Design review of the part built by this model. Coordinates are the model's own, in mm. Face numbers are marked on the shaded views. A direction names the side the tool comes from. Round coordinates to 2 decimals unless told otherwise and drop trailing zeros. Order: outer loops, then holes, each group sorted by start corner. A loop starts at its lowest first (then second) coordinate and runs counter-clockwise, first axis right, second up. Notation, with made-up numbers: (-40, -19.75) - (-25, -19.75) arc R34 cw to (-25, 16.25) - close; hole circle Ø5 at (-7.5, 51). An arc over 180 degrees is marked (long way). Write item = value, one per line.
from build123d import *

# Parameters (mm, degrees)
SKETCH_1_R                = 12
EXTRUDE_1_DEPTH           = 12
SKETCH_1_4_R              = 0.85
CUT_EXTRUDE_2_DEPTH       = 2.5
SKETCH_1_5_R              = 4
EXTRUDE_2_DEPTH           = 4
SKETCH_1_6_R              = 4.3
EXTRUDE_3_DEPTH           = 0.5
SKETCH_1_7_R              = 2
CUT_EXTRUDE_3_DEPTH       = 4
SKETCH_1_8_R              = 1.5
CUT_EXTRUDE_5_DEPTH       = 1
CUT_EXTRUDE_START         = 12
SKETCH_1_10_R             = 9
CUT_EXTRUDE_6_DEPTH       = 9.5
EXTRUDE_8_DEPTH           = 0.3
EXTRUDE_8_DEPTH_BACK      = 2.2
CUT_EXTRUDE_START_2       = -2.2
CUT_EXTRUDE_20_DEPTH      = 1.5
CUT_EXTRUDE_21_DEPTH      = 1
CUT_EXTRUDE_21_DEPTH_BACK = 2
SKETCH_3_10_R             = 0.85
FILLET_3_R                = 1.1


with BuildPart() as part:
    # 草图1 → 凸台-拉伸1 (new body)
    with BuildSketch(Plane.XY):
        Circle(SKETCH_1_R)
    extrude(amount=EXTRUDE_1_DEPTH)

    # 草图1<4> → 切除-拉伸2 (cut)
    with BuildSketch(Plane.XY):
        with Locations((0, 6)):
            Circle(SKETCH_1_4_R)
        with Locations((-5.196152423, -3)):
            Circle(SKETCH_1_4_R)
        with Locations(Location((5.196152423, -3, 0), (0, 0, 180))):
            Circle(SKETCH_1_4_R)
    extrude(amount=CUT_EXTRUDE_2_DEPTH, mode=Mode.SUBTRACT)

    # 草图1<5> → 凸台-拉伸2 (add)
    with BuildSketch(Plane.XY):
        Circle(SKETCH_1_5_R)
    extrude(amount=-EXTRUDE_2_DEPTH)

    # 草图1<6> → 凸台-拉伸3 (add)
    with BuildSketch(Plane.XY):
        Circle(SKETCH_1_6_R)
    extrude(amount=-EXTRUDE_3_DEPTH)

    # 草图1<7> → 切除-拉伸3 (cut)
    with BuildSketch(Plane.XY):
        Circle(SKETCH_1_7_R)
    extrude(amount=-CUT_EXTRUDE_3_DEPTH, mode=Mode.SUBTRACT)

    # 草图1<8> → 切除-拉伸5 (cut)
    with BuildSketch(Plane.XY):
        with Locations((-5.196152423, -3)):
            Circle(SKETCH_1_8_R)
        with Locations((5.196152423, -3)):
            Circle(SKETCH_1_8_R)
        with Locations((0, 6)):
            Circle(SKETCH_1_8_R)
    extrude(amount=CUT_EXTRUDE_5_DEPTH, mode=Mode.SUBTRACT)

    # 草图1<10> → 切除-拉伸6 (cut)
    with BuildSketch(Plane.XY.offset(CUT_EXTRUDE_START)):
        Circle(SKETCH_1_10_R)
    extrude(amount=-CUT_EXTRUDE_6_DEPTH, mode=Mode.SUBTRACT)

    # 草图3 → 凸台-拉伸8 (add, two sides: drawn at the far end of the back side and taken through both)
    with BuildSketch(Plane(origin=(14, 0, 0), x_dir=(0, 0, -1), z_dir=(1, 0, 0)).offset(-EXTRUDE_8_DEPTH_BACK)):
        Polygon((-18, -3), (-12, -3), (-6, -3), (-6, 3), (-18, 3), align=None)
        Polygon((-6, 3), (-6, -3), (0, -3), (6, -3), (6, 3), align=None)
    extrude(amount=EXTRUDE_8_DEPTH + EXTRUDE_8_DEPTH_BACK)

    # 草图3<9> → 切除-拉伸20 (cut)
    with BuildSketch(Plane(origin=(14, 0, 0), x_dir=(0, 0, -1), z_dir=(1, 0, 0)).offset(CUT_EXTRUDE_START_2)):
        Polygon((-13.130266283, 0), (-14.097327984, 1.675), (-16.031451386, 1.675), (-16.998513087, 0), (-16.031451386, -1.675), (-14.097327984, -1.675), align=None)
        Polygon((1.130266283, 0), (2.097327984, 1.675), (4.031451386, 1.675), (4.998513087, 0), (4.031451386, -1.675), (2.097327984, -1.675), align=None)
    extrude(amount=CUT_EXTRUDE_20_DEPTH, mode=Mode.SUBTRACT)

    # 草图3<10> → 切除-拉伸21 (cut, two sides: drawn at the far end of the back side and taken through both)
    with BuildSketch(Plane(origin=(14, 0, 0), x_dir=(0, 0, -1), z_dir=(1, 0, 0)).offset(-CUT_EXTRUDE_21_DEPTH_BACK)):
        with Locations(Location((3.064389685, 0, 0), (0, 0, 180))):
            Circle(SKETCH_3_10_R)
        with Locations(Location((-15.064389685, 0, 0), (0, 0, 180))):
            Circle(SKETCH_3_10_R)
    extrude(amount=CUT_EXTRUDE_21_DEPTH + CUT_EXTRUDE_21_DEPTH_BACK, mode=Mode.SUBTRACT)

    # 圆角3
    fillet_3_edges = [part.edges().sort_by_distance(p)[0] for p in [
        (13.05, 3, 18),
        (13.05, -3, 18),
        (13.05, 3, -6),
        (13.05, -3, -6),
    ]]
    fillet(fillet_3_edges, radius=FILLET_3_R)


solid = part.part
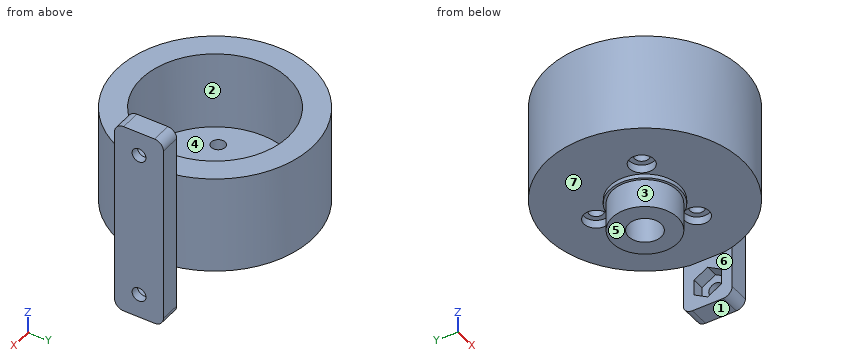
1) We need section C-C on z = 8.75. Write out the cut boundary in (x, y), and give its area (3 significant figures).
Findings:
outline = (11.8, -3) - (14.3, -3) - (14.3, 3) - (11.8, 3) - (11.8, 2.18) arc R12 ccw (long way) to (11.8, -2.18) - close; hole circle Ø18 at (0, 0)
area = 212 mm^2
2) We need section D-D on y = -10. Write out the cut boundary in (x, z).
Findings:
outline = (-6.63, 0) - (6.63, 0) - (6.63, 12) - (-6.63, 12) - close
3) Clearance check with flat-ended pins moving along their axes: pin 1 Ø1.5 at (x, y) = (0, 6.5) entering from -Z; pin 2 Ø10 at (y, z) = (-6.5, -2.5) entering from -X; pin 3 Ø4 at (x, z) = (-8, -1.5) entering from +Y. State where each tip first meets the part, or that it passes through.
Findings:
pin_1 = 1
pin_2 = -11.8
pin_3 = 9.97
4) We need section B-B on x = 8. Write out the cut boundary in (y, z), and give its area (3 significant figures).
Findings:
outline = (-8.94, 0) - (8.94, 0) - (8.94, 12) - (4.12, 12) - (4.12, 2.5) - (-4.12, 2.5) - (-4.12, 12) - (-8.94, 12) - close
area = 136 mm^2
5) To check wall thickness, follow L1, parallel to Y at x = 0, z = -0.9; L2, parallel to Y at x = 0, z = 9; L3, parallel to Z at x = 5.25, y = 6. State the ranges of each line that lie inside material, in increasing order. Write a range as from..to.
Findings:
L1 = -4..-2, 2..4
L2 = -12..-9, 9..12
L3 = 0..2.5
6) We need section A-A on y = 6. Write out the cut boundary in (x, z).
Findings:
outline = (-10.39, 0) - (-1.5, 0) - (-1.5, 1) - (-0.85, 1) - (-0.85, 2.5) - (-6.71, 2.5) - (-6.71, 12) - (-10.39, 12) - close; (0.85, 1) - (1.5, 1) - (1.5, 0) - (10.39, 0) - (10.39, 12) - (6.71, 12) - (6.71, 2.5) - (0.85, 2.5) - close
7) The part is to be moulded in two halves that separate along Y. For the marked faces 1, 2 and 3, say which applies: released by +Y, released by -Y, zero draft, split by the parting line, or undercut.
Findings:
face_1 = zero draft
face_2 = undercut
face_3 = split by the parting line
8) For the marked faces 4, 5, 6 and 7, list the 3-axis set-ups (+Z, -Z, +X, -X, +Y, -Y) from which the entire face can be reached by the end or side of a thin tool; tool diameter is ignored.
Findings:
face_4 = +Z
face_5 = -Z, -X, +Y, -Y
face_6 = none
face_7 = -Z
